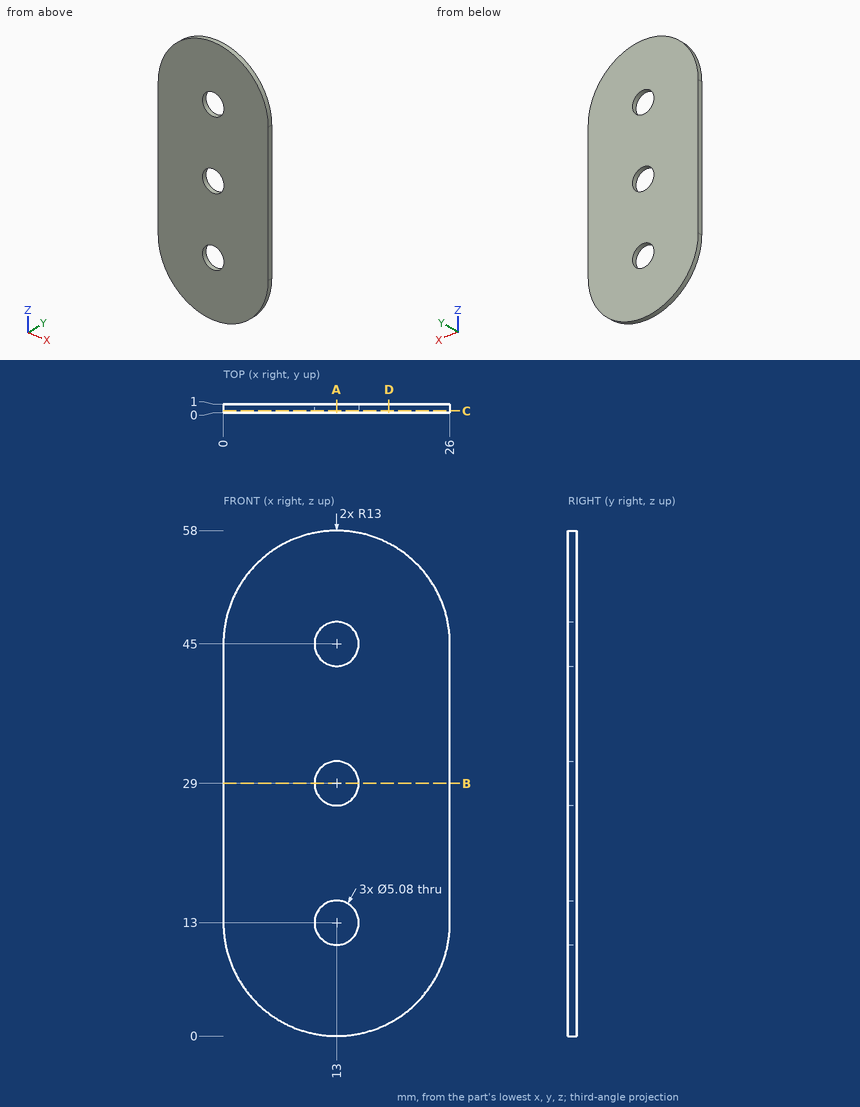
Answer from the drawing. Dimensions are ordinates in mm from the lowest x, y and z of the part. Give positions to 0.01 mm unless a question says otherwise; leave off trailing zeros. Order: outer loops, then holes, each group sorted by start corner. A loop starts at its lowest first (then second) coordinate and runs counter-clockwise, first axis right, second up. Notation, with made-up numbers: (-29.5, -13) - (13.5, -13) arc R33 cw to (13.5, 23) - close; hole circle Ø6 at (-21, 63). An arc over 180 degrees is marked (long way). One line per item, written item: value. Start each with the question number.
1) Given pin 1 Ø4.5 at (x, z) = (13, 29) entering from +Y, flat-ended and moving along its own axis, determine where the tip first touches the part or whether it passes through.
2) A cutting plane is placed at B-B on z = 29. Give the vertices of the cut face in (x, y).
3) A cutting plane is placed at D-D on x = 19. Give the vertices of the cut face in (y, z).
4) A cutting plane is placed at C-C on y = 0.2. Give the vertices of the cut face in (x, z), then the cut area to 3 significant figures.
5) A cutting plane is placed at A-A on x = 13. Give the vertices of the cut face in (y, z), then the cut area to 3 significant figures.
6) Find the intervals of material crossed by L1, parallel to Z at x = 13, y = 0.65; L2, parallel to Z at x = 10.75, y = 0.8; L3, parallel to X at y = 0.45, z = 11, in increasing order.
Answer sheet:
1. pin 1: passes through
2. outline: (0, 0) - (10.46, 0) - (10.46, 1) - (0, 1) - close; (15.54, 0) - (26, 0) - (26, 1) - (15.54, 1) - close
3. outline: (0, 1.47) - (1, 1.47) - (1, 56.53) - (0, 56.53) - close
4. outline: (0, 13) arc R13 ccw to (26, 13) - (26, 45) arc R13 ccw to (0, 45) - close; hole circle Ø5.08 at (13, 13); hole circle Ø5.08 at (13, 29); hole circle Ø5.08 at (13, 45)
4. area: 1,300 mm2
5. outline: (0, 0) - (1, 0) - (1, 10.46) - (0, 10.46) - close; (0, 15.54) - (1, 15.54) - (1, 26.46) - (0, 26.46) - close; (0, 31.54) - (1, 31.54) - (1, 42.46) - (0, 42.46) - close; (0, 47.54) - (1, 47.54) - (1, 58) - (0, 58) - close
5. area: 42.8 mm2
6. L1: z = 0 to 10.46, 15.54 to 26.46, 31.54 to 42.46, 47.54 to 58
6. L2: z = 0.2 to 11.82, 14.18 to 27.82, 30.18 to 43.82, 46.18 to 57.8
6. L3: x = 0.15 to 11.43, 14.57 to 25.85
